Part model, mm, in its own coordinate system. A direction names the side the tool comes from. Coordinates: 2 decimals unless noted, no trailing zeros. Loops run counter-clockwise (first coordinate to the right, second up) from the corner with the lowest first, then second, coordinate; pieces in that order, holes last. Notation, with made-up numbers: (-27.5, -40) - (-17.5, -40) arc R11 ccw to (-17.5, -36) - close; hole circle Ø5 at (13.5, 39). An arc over 180 degrees is marked (long way). Use a Markdown table: item, result. Add a question column.
1) Band-saw the part on B-B (x = -23). Give the cut face in (y, z).
2) Band-saw the part on C-C (y = 50). Give the cut face in (x, z), plus the area to 3 significant figures.
3) Band-saw the part on D-D (z = 79). Give the cut face in (x, y).
4) Band-saw the part on A-A (z = 28). Give the cut face in (x, y), plus the area to 3 significant figures.
5) Tool access for faces 4 (the face through (39, 79, 3)), 5 (the face through (64, -22, 51)), 6 (the face through (40, -33, 49)): list every direction of +Z, -Z, +X, -X, +Y, -Y with a clear straight run to the whole face (end or side of a thin tool).
6) Probe probe 1 along X at (y, z) = (-6.5, 79); probe 2 along Y at (x, z) = (62.5, 59.5); probe 3 along Y at (x, z) = (-27.5, 27.5). List the from-to ranges inside material, lowest first. Write a range as [from, to].
7) Pull direction X, two halves, no side cores. Call faces 1 (the face through (0, -15, 70)), 2 (the face through (77, -33, 51)), 3 (the face through (48, -30, 100)): +X half, -X half, draft (parallel to the pull), parting line (faces both ways), or undercut.
8) Drop flat-ended pins along their axis: P1, Ø2, axis at x = 53, y = 64.5, coming from the -Z side; P2, Ø6.5, axis at y = 57, z = 2.5, coming from the -X side; P3, Ø1.5, axis at x = -27, z = 4, coming from the +Y side; P4, Ø4, axis at x = 37.5, z = 22, coming from the -Y side. Give the stop position or say it passes through.
from build123d import *

# Parameters (mm, degrees)
SKETCH1_W            = 82
SKETCH1_H            = 82
BOSS_EXTRUDE1_DEPTH  = 6
SKETCH2_W            = 80
SKETCH2_H            = 80
CUT_EXTRUDE1_DEPTH   = 3
SKETCH3_W            = 82
SKETCH3_H            = 30
BOSS_EXTRUDE2_DEPTH  = 100
SKETCH4_W            = 80
SKETCH4_H            = 28
CUT_EXTRUDE2_DEPTH   = 97
SKETCH5_W            = 30
SKETCH5_H            = 30
BOSS_EXTRUDE3_DEPTH  = 40
SKETCH6_W            = 28
SKETCH6_H            = 28
CUT_EXTRUDE3_DEPTH   = 37
SKETCH7_W            = 57
SKETCH7_H            = 47
BOSS_EXTRUDE4_DEPTH  = 6
SKETCH9_W            = 55
SKETCH9_H            = 45.350877192
CUT_EXTRUDE4_DEPTH   = 3
SKETCH10_W           = 39
SKETCH10_H           = 100
BOSS_EXTRUDE6_DEPTH  = 7
SKETCH12_W           = 35
SKETCH12_H           = 5
CUT_EXTRUDE5_DEPTH   = 97
SKETCH13_W           = 55
SKETCH13_H           = 3
BOSS_EXTRUDE7_DEPTH  = 3
SKETCH14_W           = 3
SKETCH14_H           = 42.350877192
BOSS_EXTRUDE8_DEPTH  = 3
SKETCH15_W           = 6
SKETCH15_H           = 47
CUT_EXTRUDE6_DEPTH   = 3
SKETCH16_W           = 54
SKETCH16_H           = 6
CUT_EXTRUDE7_DEPTH   = 3
SKETCH17_W           = 3
SKETCH17_H           = 80
BOSS_EXTRUDE9_DEPTH  = 3
SKETCH18_W           = 77
SKETCH18_H           = 3
BOSS_EXTRUDE10_DEPTH = 3
SKETCH19_W           = 97
SKETCH19_H           = 28
BOSS_EXTRUDE11_DEPTH = 3
SKETCH20_W           = 100
SKETCH20_H           = 7
BOSS_EXTRUDE12_DEPTH = 3
SKETCH21_W           = 97
SKETCH21_H           = 5
CUT_EXTRUDE8_DEPTH   = 3
SKETCH22_W           = 97
SKETCH22_H           = 5
BOSS_EXTRUDE13_DEPTH = 3
SKETCH23_W           = 100
SKETCH23_H           = 119
CUT_EXTRUDE9_DEPTH   = 3
SKETCH24_W           = 79
SKETCH24_H           = 6
CUT_EXTRUDE10_DEPTH  = 3
SKETCH25_W           = 2
SKETCH25_H           = 28
BOSS_EXTRUDE14_DEPTH = 97
SKETCH26_W           = 13
SKETCH26_H           = 1
SKETCH26_W_2         = 1
BOSS_EXTRUDE16_DEPTH = 97
SKETCH31_W           = 97
SKETCH31_H           = 28
CUT_EXTRUDE11_DEPTH  = 1


with BuildPart() as part:
    # Sketch1 → Boss-Extrude1 (new body)
    with BuildSketch(Plane.XY):
        with Locations((41, 41)):
            Rectangle(SKETCH1_W, SKETCH1_H)
    extrude(amount=BOSS_EXTRUDE1_DEPTH)

    # Sketch2 → Cut-Extrude1 (cut)
    with BuildSketch(Plane.XY.offset(6)):
        with Locations((41, 41)):
            Rectangle(SKETCH2_W, SKETCH2_H)
    extrude(amount=-CUT_EXTRUDE1_DEPTH, mode=Mode.SUBTRACT)

    # Sketch3 → Boss-Extrude2 (add)
    with BuildSketch(Plane(origin=(0, 0, 0), x_dir=(-1, 0, 0), z_dir=(0, 0, -1))):
        with Locations((-41, -15)):
            Rectangle(SKETCH3_W, SKETCH3_H)
    extrude(amount=-BOSS_EXTRUDE2_DEPTH)

    # Sketch4 → Cut-Extrude2 (cut)
    with BuildSketch(Plane.XY.offset(100)):
        with Locations((41, -15)):
            Rectangle(SKETCH4_W, SKETCH4_H)
    extrude(amount=-CUT_EXTRUDE2_DEPTH, mode=Mode.SUBTRACT)

    # Sketch5 → Boss-Extrude3 (add)
    with BuildSketch(Plane(origin=(0, 0, 0), x_dir=(-1, 0, 0), z_dir=(0, 0, -1))):
        with Locations((15, -15)):
            Rectangle(SKETCH5_W, SKETCH5_H)
    extrude(amount=-BOSS_EXTRUDE3_DEPTH)

    # Sketch6 → Cut-Extrude3 (cut)
    with BuildSketch(Plane.XY.offset(40)):
        with Locations((-15, -15)):
            Rectangle(SKETCH6_W, SKETCH6_H)
    extrude(amount=-CUT_EXTRUDE3_DEPTH, mode=Mode.SUBTRACT)

    # Sketch7 → Boss-Extrude4 (add)
    with BuildSketch(Plane(origin=(0, 0, 0), x_dir=(-1, 0, 0), z_dir=(0, 0, -1))):
        with Locations((28.5, 23.5)):
            Rectangle(SKETCH7_W, SKETCH7_H)
    extrude(amount=-BOSS_EXTRUDE4_DEPTH)

    # Sketch9 → Cut-Extrude4 (cut)
    with BuildSketch(Plane.XY.offset(6)):
        with Locations((-28.5, 23.5)):
            Rectangle(SKETCH9_W, SKETCH9_H)
    extrude(amount=-CUT_EXTRUDE4_DEPTH, mode=Mode.SUBTRACT)

    # Sketch10 → Boss-Extrude6 (add)
    with BuildSketch(Plane(origin=(0, -30, 0), x_dir=(-1, 0, 0), z_dir=(0, -1, 0))):
        with Locations((-62.5, -50)):
            Rectangle(SKETCH10_W, SKETCH10_H)
    extrude(amount=BOSS_EXTRUDE6_DEPTH)

    # Sketch12 → Cut-Extrude5 (cut)
    with BuildSketch(Plane.XY.offset(100)):
        with Locations((62.5, -33)):
            Rectangle(SKETCH12_W, SKETCH12_H)
    extrude(amount=-CUT_EXTRUDE5_DEPTH, mode=Mode.SUBTRACT)

    # Sketch13 → Boss-Extrude7 (add)
    with BuildSketch(Plane.XZ.offset(-46.175438596)):
        with Locations((-28.5, 4.5)):
            Rectangle(SKETCH13_W, SKETCH13_H)
    extrude(amount=BOSS_EXTRUDE7_DEPTH)

    # Sketch14 → Boss-Extrude8 (add)
    with BuildSketch(Plane(origin=(-56, 0, 0), x_dir=(0, 0, -1), z_dir=(1, 0, 0))):
        with Locations((-4.5, 22)):
            Rectangle(SKETCH14_W, SKETCH14_H)
    extrude(amount=BOSS_EXTRUDE8_DEPTH)

    # Sketch15 → Cut-Extrude6 (cut)
    with BuildSketch(Plane.ZY.offset(57)):
        with Locations((3, 23.5)):
            Rectangle(SKETCH15_W, SKETCH15_H)
    extrude(amount=-CUT_EXTRUDE6_DEPTH, mode=Mode.SUBTRACT)

    # Sketch16 → Cut-Extrude7 (cut)
    with BuildSketch(Plane(origin=(0, 47, 0), x_dir=(1, 0, 0), z_dir=(0, 1, 0))):
        with Locations((-27, -3)):
            Rectangle(SKETCH16_W, SKETCH16_H)
    extrude(amount=-CUT_EXTRUDE7_DEPTH, mode=Mode.SUBTRACT)

    # Sketch17 → Boss-Extrude9 (add)
    with BuildSketch(Plane.ZY.offset(-81)):
        with Locations((4.5, 41)):
            Rectangle(SKETCH17_W, SKETCH17_H)
    extrude(amount=BOSS_EXTRUDE9_DEPTH)

    # Sketch18 → Boss-Extrude10 (add)
    with BuildSketch(Plane.XZ.offset(-81)):
        with Locations((39.5, 4.5)):
            Rectangle(SKETCH18_W, SKETCH18_H)
    extrude(amount=BOSS_EXTRUDE10_DEPTH)

    # Sketch19 → Boss-Extrude11 (add)
    with BuildSketch(Plane.ZY.offset(-81)):
        with Locations((51.5, -15)):
            Rectangle(SKETCH19_W, SKETCH19_H)
    extrude(amount=BOSS_EXTRUDE11_DEPTH)

    # Sketch20 → Boss-Extrude12 (add)
    with BuildSketch(Plane.ZY.offset(-43)):
        with Locations((50, -33.5)):
            Rectangle(SKETCH20_W, SKETCH20_H)
    extrude(amount=BOSS_EXTRUDE12_DEPTH)

    # Sketch21 → Cut-Extrude8 (cut)
    with BuildSketch(Plane(origin=(45, 0, 0), x_dir=(0, 0, -1), z_dir=(1, 0, 0))):
        with Locations((-51.5, -33)):
            Rectangle(SKETCH21_W, SKETCH21_H)
    extrude(amount=-CUT_EXTRUDE8_DEPTH, mode=Mode.SUBTRACT)

    # Sketch22 → Boss-Extrude13 (add)
    with BuildSketch(Plane.ZY.offset(-80)):
        with Locations((51.5, -33)):
            Rectangle(SKETCH22_W, SKETCH22_H)
    extrude(amount=BOSS_EXTRUDE13_DEPTH)

    # Sketch23 → Cut-Extrude9 (cut)
    with BuildSketch(Plane(origin=(82, 0, 0), x_dir=(0, 0, -1), z_dir=(1, 0, 0))):
        with Locations((-50, 22.5)):
            Rectangle(SKETCH23_W, SKETCH23_H)
    extrude(amount=-CUT_EXTRUDE9_DEPTH, mode=Mode.SUBTRACT)

    # Sketch24 → Cut-Extrude10 (cut)
    with BuildSketch(Plane(origin=(0, 82, 0), x_dir=(1, 0, 0), z_dir=(0, 1, 0))):
        with Locations((39.5, -3)):
            Rectangle(SKETCH24_W, SKETCH24_H)
    extrude(amount=-CUT_EXTRUDE10_DEPTH, mode=Mode.SUBTRACT)

    # Sketch25 → Boss-Extrude14 (add)
    with BuildSketch(Plane.XY.offset(3)):
        with Locations((63, -15)):
            Rectangle(SKETCH25_W, SKETCH25_H)
    extrude(amount=BOSS_EXTRUDE14_DEPTH)

    # Sketch26 → Boss-Extrude16 (add)
    with BuildSketch(Plane.XY.offset(3)):
        with Locations((70.5, -15)):
            Rectangle(SKETCH26_W, SKETCH26_H)
        with Locations((77.5, -15)):
            Rectangle(SKETCH26_W_2, SKETCH26_H)
    extrude(amount=BOSS_EXTRUDE16_DEPTH)

    # Sketch31 → Cut-Extrude11 (cut)
    with BuildSketch(Plane.ZY.offset(-62)):
        with Locations((51.5, -15)):
            Rectangle(SKETCH31_W, SKETCH31_H)
    extrude(amount=-CUT_EXTRUDE11_DEPTH, mode=Mode.SUBTRACT)


solid = part.part
Answer block:
| question | item | result |
|---|---|---|
| 1 | outline | (-30, 0) - (44, 0) - (44, 6) - (43.18, 6) - (43.18, 3) - (0.82, 3) - (0.82, 6) - (0, 6) - (0, 40) - (-1, 40) - (-1, 3) - (-29, 3) - (-29, 40) - (-30, 40) - close |
| 2 | outline | (0, 0) - (79, 0) - (79, 6) - (78, 6) - (78, 3) - (1, 3) - (1, 6) - (0, 6) - close |
| 2 | area | 243 mm2 |
| 3 | outline | (0, -30) - (40, -30) - (40, -37) - (79, -37) - (79, 0) - (0, 0) - close; hole (1, -29) - (63, -29) - (63, -1) - (1, -1) - close; hole (42, -35.5) - (77, -35.5) - (77, -30.5) - (42, -30.5) - close; hole (64, -29) - (78, -29) - (78, -15.5) - (64, -15.5) - close; hole (64, -14.5) - (78, -14.5) - (78, -1) - (64, -1) - close |
| 4 | outline | (-30, -30) - (40, -30) - (40, -37) - (79, -37) - (79, 0) - (-30, 0) - close; hole (-29, -29) - (-1, -29) - (-1, -1) - (-29, -1) - close; hole (1, -29) - (63, -29) - (63, -1) - (1, -1) - close; hole (42, -35.5) - (77, -35.5) - (77, -30.5) - (42, -30.5) - close; hole (64, -29) - (78, -29) - (78, -15.5) - (64, -15.5) - close; hole (64, -14.5) - (78, -14.5) - (78, -1) - (64, -1) - close |
| 4 | area | 470 mm2 |
| 5 | face 4 | +Z, -Z, +X, -X, +Y |
| 5 | face 5 | +Z |
| 5 | face 6 | +Z, -Z, -X, -Y |
| 6 | probe 1 | [0, 1], [63, 64], [78, 79] |
| 6 | probe 2 | [-37, -35.5], [-30.5, -29], [-1, 0] |
| 6 | probe 3 | [-30, -29], [-1, 0] |
| 7 | face 1 | -X half |
| 7 | face 2 | undercut |
| 7 | face 3 | draft |
| 8 | P1 | z = 0 |
| 8 | P2 | x = 0 |
| 8 | P3 | y = 44 |
| 8 | P4 | y = -30 |
